The listing builds one solid part. Answer for the finished solid, in the listing's coordinates (mm). Face numbers are marked on the shaded views. Round coordinates to 2 decimals unless told otherwise and drop trailing zeros. Loops run counter-clockwise (first coordinate to the right, second up) from the corner with the lowest first, then second, coordinate; pieces in that order, holes last. Notation, with made-up numbers: M -28.5,3 L -1.5,3 A13 ccw -1.5,12 Z; hole C 18.5,-10.75 d11. An arc over 180 degrees is marked long. Put each result on its own line as item: value. Start each with the question number.
(1) Section A-A, the plane y = 25.5 is taken. Determine the outline of the cut face in (x, z), then the cut area to 3 significant figures.
(2) Straight lines are drawn through the part: line 1 (Y direction, x = 17, z = -18.5); line 2 (Z direction, x = 19.5, y = 14); line 3 (Z direction, x = 5.5, y = 3.5). For each, find the intervals that lie inside material, in ascending order.
(3) Flat-ended cylindrical pins translate along their axes: P1, Ø12, axis at y = 19, z = -49, coming from the +X side; P2, Ø10, axis at x = 27, y = 7, coming from the -Z side; P3, Ø12, axis at x = 16, z = -13, coming from the -Y side. Find the tip coordinate at first contact, or state that the pin passes through.
(4) Determine the mould class of the marked faces 1, 2 and 3 for opening direction X: released by +X, released by -X, zero draft, split by the parting line, or undercut.
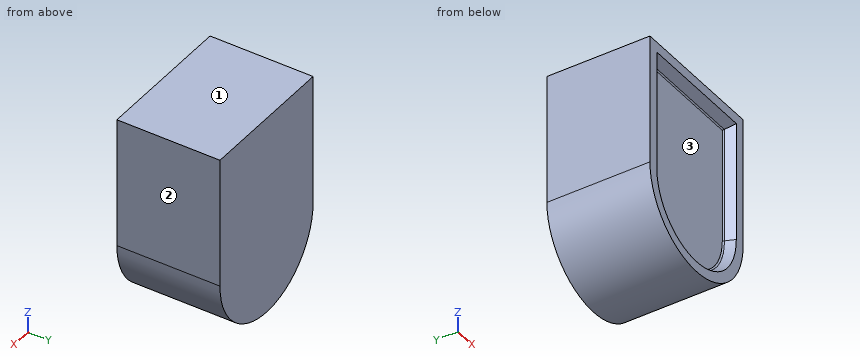
```python
from build123d import *

# Parameters (mm, degrees)
SKETCH2_W           = 35
SKETCH2_H           = 35
BOSS_EXTRUDE1_DEPTH = 30
FILLET1_R           = 0.5


with BuildPart() as part:
    # Sketch2 → Boss-Extrude1 (new body)
    with BuildSketch(Plane(origin=(0, 0, 0), x_dir=(1, 0, 0), z_dir=(0, 1, 0))):
        Polygon((35, 0), (0, 0), (0, 35), (-3, 35), (-3, 0), (-3, -3), (38, -3), (38, 0), (38, 35), (35, 35), align=None)
        with BuildLine():
            Line((-3, 35), (0, 35))
            ThreePointArc((0, 35), (17.5, 52.5), (35, 35))
            Line((35, 35), (38, 35))
            ThreePointArc((38, 35), (17.5, 55.5), (-3, 35))
        make_face()
        with Locations((17.5, 17.5)):
            Rectangle(SKETCH2_W, SKETCH2_H)
        with BuildLine():
            ThreePointArc((35, 35), (17.5, 52.5), (0, 35))
            Line((0, 35), (35, 35))
        make_face()
    extrude(amount=BOSS_EXTRUDE1_DEPTH)

    # Sketch2_9 → Cut-Loft1 section 0
    with BuildSketch(Plane(origin=(0, 0, 0), x_dir=(1, 0, 0), z_dir=(0, 1, 0))):
        with BuildLine():
            Line((0, 0), (0, 35))
            ThreePointArc((0, 35), (17.5, 52.5), (35, 35))
            Line((35, 35), (35, 0))
            Line((35, 0), (0, 0))
        make_face()
    # Sketch3 → Cut-Loft1 section 1
    with BuildSketch(Plane(origin=(0, 3.02, 0), x_dir=(-1, 0, 0), z_dir=(0, -1, 0))):
        with BuildLine():
            Line((-33.75, 1.5), (-1.25, 1.5))
            Line((-1.25, 1.5), (-1.25, 35))
            ThreePointArc((-1.25, 35), (-17.5, 51.25), (-33.75, 35))
            Line((-33.75, 35), (-33.75, 1.5))
        make_face()
    loft(mode=Mode.SUBTRACT)

    # Fillet1
    fillet1_edges = [part.edges().sort_by_distance(p)[0] for p in [
        (1.25, 3.02, -18.25),
        (33.75, 3.02, -18.25),
        (17.5, 3.02, -1.5),
        (17.5, 3.02, -51.25),
    ]]
    fillet(fillet1_edges, radius=FILLET1_R)


solid = part.part
```
Recorded:
1. outline: M -3,-35 A20.5 ccw 38,-35 L 38,3 L -3,3 Z
1. area: 2,220 mm²
2. line 1: y = 3.02 to 30
2. line 2: z = -55.4 to 3
2. line 3: z = -51.62 to 3
3. P1: stops at x = 36.37
3. P2: stops at z = -55
3. P3: stops at y = 3.02
4. face 1: zero draft
4. face 2: released by +X
4. face 3: undercut
